The model under review builds one solid part; all positions refer to its coordinate system, in mm. Round coordinates to 2 decimals unless told otherwise and drop trailing zeros. Order: outer loops, then holes, each group sorted by start corner. A loop starts at its lowest first (then second) coordinate and runs counter-clockwise, first axis right, second up. Notation, with made-up numbers: (13, 63) -> (40, 63) arc R27 ccw to (40, 101) -> close; hole circle Ø5 at (-2, 44.25). An arc over 180 degrees is marked (long way). Return JSON: item names as keys, results as strings. Group by question number.
from build123d import *

# Parameters (mm, degrees)
COCKPIT_TEMPLATE_DEPTH = 304.8


with BuildPart() as part:
    # Sketch11 → Cockpit Template (new, symmetric)
    with BuildSketch(Plane.XY.offset(1043.931203382)):
        with BuildLine():
            Line((125, 468.656673601), (50, 468.656673601))
            ThreePointArc((50, 468.656673601), (0, 418.656673601), (-50, 468.656673601))
            Line((-50, 468.656673601), (-125, 468.656673601))
            Line((-125, 468.656673601), (-175, 418.656673601))
            Line((-175, 418.656673601), (-175, 168.656673601))
            Line((-175, 168.656673601), (-125, 118.656673601))
            Line((-125, 118.656673601), (-50, 118.656673601))
            ThreePointArc((-50, 118.656673601), (0, 168.656673601), (50, 118.656673601))
            Line((50, 118.656673601), (125, 118.656673601))
            Line((125, 118.656673601), (175, 168.656673601))
            Line((175, 168.656673601), (175, 418.656673601))
            Line((175, 418.656673601), (125, 468.656673601))
        make_face()
    extrude(amount=COCKPIT_TEMPLATE_DEPTH, both=True)


solid = part.part
Item 1: Wall thickness on line 1 along Y through (x, z) = (-1.5, 1019); line 2 along X through (y, z) = (444, 905); line 3 along Y through (x, z) = (40, 895.5): over which ranges is each line inside the solid? List them lowest first.
Item 2: Consider section B-B on x = 0. State the section outline as (y, z) points, plus the area to 3 significant figures.
Item 3: The part is to be moulded in two halves that separate along X. For faces 1 (the face through (-1.099, 168.645, 1048.198)), 2 (the face through (-2, 296, 1348.731)), 3 (the face through (-150.35, 144.007, 1048.198)), say which applies: +X half, -X half, draft (parallel to the pull), parting line (faces both ways), or undercut.
Item 4: Consider section C-C on x = 144.5. State the section outline as (y, z) points, plus the area to 3 significant figures.
Item 5: Consider section A-A on z = 1221.5. State the section outline as (x, y) points.
Values:
{
 "1": {"line 1": "168.63 to 418.68", "line 2": "-149.66 to -43.5, 43.5 to 149.66", "line 3": "148.66 to 438.66"},
 "2": {"outline": "(168.66, 739.13) -> (418.66, 739.13) -> (418.66, 1348.73) -> (168.66, 1348.73) -> close", "area": "152,000 mm^2"},
 "3": {"face 1": "undercut", "face 2": "draft", "face 3": "-X half"},
 "4": {"outline": "(138.16, 739.13) -> (449.16, 739.13) -> (449.16, 1348.73) -> (138.16, 1348.73) -> close", "area": "190,000 mm^2"},
 "5": {"outline": "(-175, 168.66) -> (-125, 118.66) -> (-50, 118.66) arc R50 cw to (50, 118.66) -> (125, 118.66) -> (175, 168.66) -> (175, 418.66) -> (125, 468.66) -> (50, 468.66) arc R50 cw to (-50, 468.66) -> (-125, 468.66) -> (-175, 418.66) -> close"}
}
